from build123d import *

# Parameters (mm, degrees)
BOSS_EXTRU_1_DEPTH           = 25
ENL_V_MAT_EXTRU_2_DEPTH      = 58.853262656
ENL_V_MAT_EXTRU_2_DEPTH_BACK = 58.853262656
BOSS_EXTRU_2_DEPTH           = 1.5
CONG_1_R                     = 5


with BuildPart() as part:
    # Esquisse1 → Boss.-Extru.1 (new body)
    with BuildSketch(Plane(origin=(0, 0, 0), x_dir=(1, 0, 0), z_dir=(0, 1, 0))):
        with BuildLine():
            Line((0.76744186, 10.973196116), (43.558139535, 7.980506266))
            ThreePointArc((43.558139535, 7.980506266), (51, 0), (43.558139535, -7.980506266))
            Line((43.558139535, -7.980506266), (0.76744186, -10.973196116))
            ThreePointArc((0.76744186, -10.973196116), (-11, 0), (0.76744186, 10.973196116))
        make_face()
        with BuildLine():
            Line((43, -3.5), (38, -3.5))
            ThreePointArc((38, -3.5), (34.5, 0), (38, 3.5))
            Line((38, 3.5), (43, 3.5))
            ThreePointArc((43, 3.5), (46.5, 0), (43, -3.5))
        make_face(mode=Mode.SUBTRACT)
    extrude(amount=BOSS_EXTRU_1_DEPTH)

    # Esquisse4 → Enlèv. mat.-Extru.2 (cut, two sides: drawn at the far end of the back side and taken through both)
    with BuildSketch(Plane.XY.offset(-ENL_V_MAT_EXTRU_2_DEPTH_BACK)):
        Polygon((-11, 0), (28.567731326, 0), (15, 23.5), (-11, 23.5), align=None)
        Polygon((51, 25), (15.866025404, 25), (27.990381057, 4), (51, 4), align=None)
    extrude(amount=ENL_V_MAT_EXTRU_2_DEPTH + ENL_V_MAT_EXTRU_2_DEPTH_BACK, mode=Mode.SUBTRACT)

    # Esquisse6 → Boss.-Extru.2 (add)
    with BuildSketch(Plane(origin=(0.76744186, 0, 10.973196116), x_dir=(0.997563283233824, 0, -0.0697674418604651), z_dir=(0.0697674418604651, 0, 0.9975632832338241))):
        Polygon((9.645698279, 25), (18.888948853, 25), (33.357962471, 0), (24.114711897, 0), align=None)
    boss_extru_2 = extrude(amount=-BOSS_EXTRU_2_DEPTH)

    # Symétrie1: Boss.-Extru.2 across plane
    add(boss_extru_2.mirror(Plane.XY))

    # Congé1
    cong_1_edges = [part.edges().sort_by_distance(p)[0] for p in [
        (27.990381057, 4, 0),
        (15, 23.5, 0),
        (28.567731326, 0, 0),
        (15.866025404, 25, 0),
        (24.771067454, 0, -8.542601893),
        (19.558038113, 25, -8.907190012),
        (24.771067454, 0, 8.542601893),
        (19.558038113, 25, 8.907190012),
    ]]
    fillet(cong_1_edges, radius=CONG_1_R)


solid = part.part
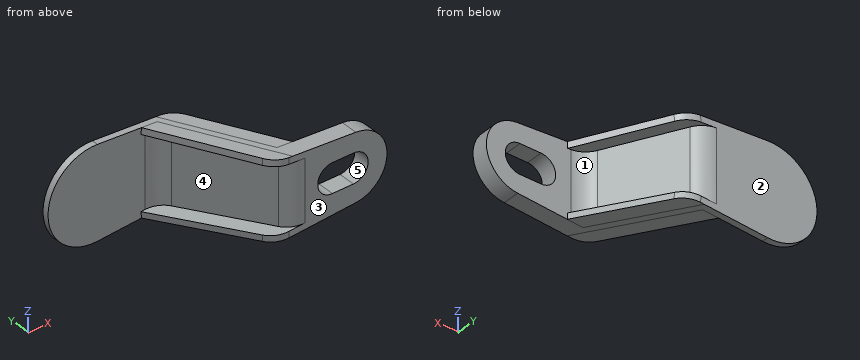
Can you work these out from the model? Positions are in its coordinate system, mm. Face numbers are marked on the shaded views. A direction names the side the tool comes from. Round coordinates to 2 decimals unless told otherwise and drop trailing zeros. Loops run counter-clockwise (first coordinate to the right, second up) from the corner with the lowest first, then second, coordinate; pieces in that order, holes last. Notation, with made-up numbers: (-34, 17.5) - (11, 17.5) arc R20 ccw to (11, 55.5) - close; hole circle Ø4 at (15.5, 44). An arc over 180 degrees is marked (long way). Answer in a Markdown table with one row per item. Add a question column.
Q1. I want a section at B-B on x = 39.5. List the corners of the cut face in (y, z) for me, and give its area (3 significant figures).
Q2. I want a section at D-D on z = -5. List the corners of the cut face in (x, y) for me (3 decimals).
Q3. For pin 1 Ø2 at (x, y) = (41, 1.5) entering from -Z; pin 2 Ø12 at (x, z) = (5.5, -8) entering from -Y; pin 3 Ø2 at (x, z) = (19, -2) entering from -Y, each with a flat end and sliding along its axis, tell me the tip position at first contact or that it passes through.
Q4. I want a section at A-A on z = 0. List the corners of the cut face in (x, y) for me.
Q5. I want a section at C-C on y = 7.75. List the corners of the cut face in (x, z) for me (3 decimals).
Q6. We'd pull the mould along Z, two halves only. Please class the marked faces 1 and 2: pulls with the +Z half, pulls with the -Z half, needs draft (parallel to the pull), parting line crosses it, or undercut.
Q7. Which directions (+Z, -Z, +X, -X, +Y, -Y) give clear straight access to the entire face, cutting with the end or side of a thin tool? Please do the marked faces 3, 4 and 5.
Q8. I need wall thicknesses on L1, parallel to Z at x = 21, y = 11.75; L2, parallel to Y at x = -2, z = 0.75; L3, parallel to Y at x = 33.5, z = 2. Which ranges of each line are inside material? Lowest first, please.
A:
| question | item | result |
|---|---|---|
| 1 | outline | (0, -8.26) - (4, -8.26) - (4, -3.5) - (0, -3.5) - close; (0, 3.5) - (4, 3.5) - (4, 8.26) - (0, 8.26) - close |
| 1 | area | 38.1 mm^2 |
| 2 | outline | (-9.798, 23.5) - (12.113, 23.5) arc R5 cw to (16.443, 21) - (27.124, 2.5) arc R5 ccw to (31.454, 0) - (49.245, 0) - (49.245, 4) - (30.877, 4) arc R5 cw to (26.547, 6.5) - (17.309, 22.5) arc R5 ccw to (12.979, 25) - (-9.798, 25) - close |
| 3 | pin 1 | z = -8.23 |
| 3 | pin 2 | y = 22.97 |
| 3 | pin 3 | y = 14.84 |
| 4 | outline | (-11, 23.5) - (12.11, 23.5) arc R5 cw to (16.44, 21) - (27.12, 2.5) arc R5 ccw to (31.45, 0) - (34.5, 0) - (34.5, 4) - (30.88, 4) arc R5 cw to (26.55, 6.5) - (17.31, 22.5) arc R5 ccw to (12.98, 25) - (-11, 25) - close; (46.5, 0) - (51, 0) - (51, 4) - (46.5, 4) - close |
| 5 | outline | (20.244, -8.107) - (20.349, -9.604) - (29.57, -8.959) - (29.465, -7.462) - (25.825, -7.717) - (25.825, 7.717) - (29.465, 7.462) - (29.57, 8.959) - (20.349, 9.604) - (20.244, 8.107) - (24.093, 7.838) - (24.093, -7.838) - close |
| 6 | face 1 | undercut |
| 6 | face 2 | needs draft |
| 7 | face 3 | +Z, -Z, +X, -X, -Y |
| 7 | face 4 | -X, -Y |
| 7 | face 5 | +Y, -Y |
| 8 | L1 | -9.56 to -8.05, 8.05 to 9.56 |
| 8 | L2 | 23.5 to 25 |
| 8 | L3 | 0 to 4 |
